The model under review builds one solid part; all positions refer to its coordinate system, in mm. A direction names the side the tool comes from. Round coordinates to 2 decimals unless told otherwise and drop trailing zeros. Write each loop counter-clockwise with the first axis right and the second up, starting at its lowest first coordinate (ties: lowest second). Pieces come first, ordered by that corner, then holes. Notation, with made-up numbers: M 55.5,62 L 99.5,62 A27 ccw 99.5,91 Z; hole C 25,36.25 d6. An arc over 180 degrees is marked long. Write item = value, one per line. Start each with the question number.
Item 1: Take a section at D-D, the plane x = 7. Give the boundary of the cut face in (y, z).
Item 2: Take a section at A-A, the plane y = 0. Give the number of separate pieces and of enclosed holes in the cut face, plus the area to 3 significant figures.
Item 3: Take a section at C-C, the plane y = 7. Give the boundary of the cut face in (x, z).
Item 4: Take a section at B-B, the plane x = 0. Give the boundary of the cut face in (y, z), plus the area to 3 significant figures.
Item 5: To check wall thickness, follow line 1 along X through (y, z) = (1, 9); line 2 along Y through (x, z) = (-10, 3.95); line 3 along Y through (x, z) = (-10, 1.45). State the ranges of each line that lie inside material, in increasing order.
Item 6: For pin 1 Ø1 at (x, y) = (13.5, 1) entering from -Z; pin 2 Ø7 at (x, y) = (10, 0) entering from +Z; pin 3 Ø7 at (x, z) = (0, 5.89) entering from -Y, all flat-tipped, find the tip position at first contact; note any pin that passes through.
Item 7: Tool access review of faces 1 (the flat face through (8, -2, 2)), 2 (the flat face through (-8.08, -3.39, 9.54)), 3 (the flat face through (0, 0, 0)): name each direction out of +Z, -Z, +X, -X, +Y, -Y from which nothing blocks a thin tool from reaching the whole face with its end or side.
Item 8: The part is to be moulded in two halves that separate along Z. For faces 4 (the flat face through (-12, -2, 7)), 5 (the cylindrical face through (-1.149, 0.112, 8.664)), 6 (the flat face through (-0.2, -10, 11.2)), 7 (the flat face through (-12, -2, 2)), say which applies: +Z half, -Z half, draft (parallel to the pull), parting line (faces both ways), or undercut.
from build123d import *

# Parameters (mm, degrees)
SKETCH1_W           = 34
SKETCH1_H           = 20
BOSS_EXTRUDE1_DEPTH = 12
SKETCH2_R           = 2.5
CUT_EXTRUDE5_DEPTH  = 12
SKETCH2_8_R         = 4.3
SKETCH2_8_R_2       = 2.5
CUT_EXTRUDE6_DEPTH  = 2
SKETCH6_R           = 3
CUT_EXTRUDE7_DEPTH  = 20
FILLET1_R           = 2
CUT_EXTRUDE8_DEPTH  = 5


with BuildPart() as part:
    # Sketch1 → Boss-Extrude1 (new body)
    with BuildSketch(Plane.XY):
        Rectangle(SKETCH1_W, SKETCH1_H)
    extrude(amount=BOSS_EXTRUDE1_DEPTH)

    # Sketch2 → Cut-Extrude5 (cut)
    with BuildSketch(Plane(origin=(0, 0, 0), x_dir=(-1, 0, 0), z_dir=(0, 0, -1))):
        with Locations((10, 0)):
            Circle(SKETCH2_R)
        with Locations((-10, 0)):
            Circle(SKETCH2_R)
    extrude(amount=-CUT_EXTRUDE5_DEPTH, mode=Mode.SUBTRACT)

    # Sketch2<8> → Cut-Extrude6 (cut)
    # profile 1 of 2: a face of its own
    with BuildSketch(Plane(origin=(0, 0, 0), x_dir=(-1, 0, 0), z_dir=(0, 0, -1))):
        with Locations((10, 0)):
            Circle(SKETCH2_8_R)
        with Locations((10, 0)):
            Circle(SKETCH2_8_R_2, mode=Mode.SUBTRACT)
    # profile 2 of 2: a face of its own
    with BuildSketch(Plane(origin=(0, 0, 0), x_dir=(-1, 0, 0), z_dir=(0, 0, -1))):
        with Locations((-10, 0)):
            Circle(SKETCH2_8_R)
        with Locations((-10, 0)):
            Circle(SKETCH2_8_R_2, mode=Mode.SUBTRACT)
    extrude(amount=-CUT_EXTRUDE6_DEPTH, mode=Mode.SUBTRACT)

    # Sketch6 → Cut-Extrude7 (cut)
    with BuildSketch(Plane(origin=(0, 10, 0), x_dir=(1, 0, 0), z_dir=(0, 1, 0))):
        with Locations(Location((0, -5.892499296, 0), (0, 0, 270))):
            Circle(SKETCH6_R)
    extrude(amount=-CUT_EXTRUDE7_DEPTH, mode=Mode.SUBTRACT)

    # Fillet1
    fillet1_edges = [part.edges().sort_by_distance(p)[0] for p in [
        (0, 10, 2.892499296),
        (0, -10, 2.892499296),
    ]]
    fillet(fillet1_edges, radius=FILLET1_R)

    # Sketch7 → Cut-Extrude8 (cut)
    with BuildSketch(Plane.XY.offset(12)):
        Polygon((-10, 4.5), (-13.897114317, 2.25), (-13.897114317, -2.25), (-10, -4.5), (-6.102885683, -2.25), (-6.102885683, 2.25), align=None)
        Polygon((10, 4.5), (6.102885683, 2.25), (6.102885683, -2.25), (10, -4.5), (13.897114317, -2.25), (13.897114317, 2.25), align=None)
    extrude(amount=-CUT_EXTRUDE8_DEPTH, mode=Mode.SUBTRACT)


solid = part.part
Response values:
q1.outline = M -10,0 L -3.08,0 L -3.08,2 L 3.08,2 L 3.08,0 L 10,0 L 10,12 L 2.77,12 L 2.77,7 L -2.77,7 L -2.77,12 L -10,12 Z
q2.separate_pieces = 3
q2.enclosed_holes = 1
q2.area = 217 mm2
q3.outline = M -17,0 L 17,0 L 17,12 L -17,12 Z; hole C 0,5.89 d6
q4.outline = M -10,0 L 10,0 L 10,0.89 A2 ccw 8,2.89 L -8,2.89 A2 ccw -10,0.89 Z; M -10,10.89 A2 ccw -8,8.89 L 8,8.89 A2 ccw 10,10.89 L 10,12 L -10,12 Z
q4.area = 117 mm2
q5.line_1 = -17 to -13.9, -6.1 to 6.1, 13.9 to 17
q5.line_2 = -10 to -2.5, 2.5 to 10
q5.line_3 = -10 to -4.3, 4.3 to 10
q6.pin_1 = 2
q6.pin_2 = 7
q6.pin_3 = -9.33
q7.face_1 = -Z
q7.face_2 = +Z
q7.face_3 = -Z, +X, -X, +Y, -Y
q8.face_4 = +Z half
q8.face_5 = undercut
q8.face_6 = draft
q8.face_7 = -Z half
